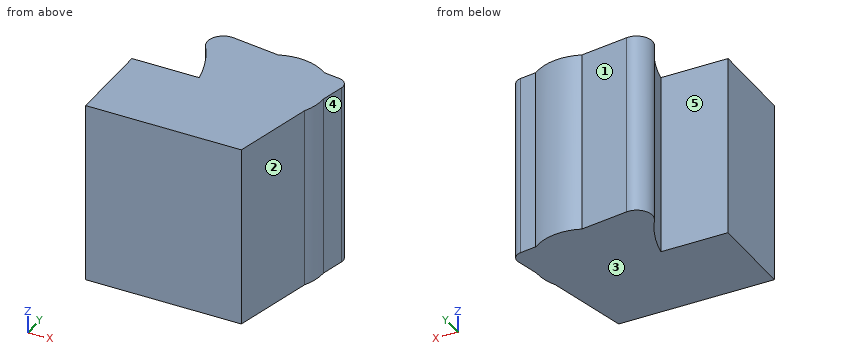
```python
from build123d import *

# Parameters (mm, degrees)
SKETCH_1_R                     = 27.60110162
EXTRUDE_1_DEPTH                = 50
SPLIT_BODIES_1_SURFACE_1_BACK  = 231.64
SPLIT_BODIES_1_SURFACE_1_DEPTH = 463.28
SPLIT_BODIES_1_SURFACE_2_BACK  = 231.64
SPLIT_BODIES_1_SURFACE_2_DEPTH = 463.28


with BuildPart() as part:
    # 草图1 → 凸台-拉伸1 (new, symmetric)
    with BuildSketch(Plane.XY):
        with Locations((126.841, 106.3205)):
            Circle(SKETCH_1_R)
        with BuildLine():
            Line((0, 29.556947787), (33.841128496, 29.556947787))
            Line((33.841128496, 29.556947787), (55.404404979, 43.133825573))
            Line((55.404404979, 43.133825573), (55.404404979, 95.897124924))
            Line((55.404404979, 95.897124924), (92.202864513, 95.897124924))
            ThreePointArc((92.202864513, 95.897124924), (88.266951773, 109.605982584), (81.786119565, 122.311217777))
            ThreePointArc((81.786119565, 122.311217777), (81.790702408, 131.54578908), (90.169806602, 135.427533672))
            Line((90.169806602, 135.427533672), (152.632483554, 126.981321854))
            ThreePointArc((152.632483554, 126.981321854), (156.573746893, 124.561834969), (157.437634447, 120.018579331))
            Line((157.437634447, 120.018579331), (140.698476255, 47.962391292))
            Line((140.698476255, 47.962391292), (125.156200351, 47.962391292))
            Line((125.156200351, 47.962391292), (116.770080258, 26.493923855))
            Line((116.770080258, 26.493923855), (133.542320443, 26.493923855))
            Line((133.542320443, 26.493923855), (144.001, 0))
            Line((144.001, 0), (0, 0))
            Line((0, 0), (0, 29.556947787))
        make_face()
    extrude(amount=EXTRUDE_1_DEPTH, both=True)


with BuildPart() as body_2:
    # Split Bodies 1: the piece behind the surface
    add(part.part)
    # Split Bodies 1 surface: a surface, the sketch's curves swept straight by 463.28 mm
    with BuildLine(Plane.XY.offset(50).offset(-SPLIT_BODIES_1_SURFACE_1_BACK), mode=Mode.PRIVATE) as split_bodies_1_surface_1_path:
        Line((125.156200351, 47.962391292), (37.921543342, 47.962391292))
    split_bodies_1_surface_1 = Shell.extrude(split_bodies_1_surface_1_path.wire(), (0 * SPLIT_BODIES_1_SURFACE_1_DEPTH, 0 * SPLIT_BODIES_1_SURFACE_1_DEPTH, 1 * SPLIT_BODIES_1_SURFACE_1_DEPTH))
    split(bisect_by=split_bodies_1_surface_1, keep=Keep.BOTTOM)


with BuildPart() as part_1:
    add(part.part)

    # Split Bodies 1: split by a surface, the side it looks to stays
    # Split Bodies 1 surface: a surface, the sketch's curves swept straight by 463.28 mm
    with BuildLine(Plane.XY.offset(50).offset(-SPLIT_BODIES_1_SURFACE_2_BACK), mode=Mode.PRIVATE) as split_bodies_1_surface_2_path:
        Line((125.156200351, 47.962391292), (37.921543342, 47.962391292))
    split_bodies_1_surface_2 = Shell.extrude(split_bodies_1_surface_2_path.wire(), (0 * SPLIT_BODIES_1_SURFACE_2_DEPTH, 0 * SPLIT_BODIES_1_SURFACE_2_DEPTH, 1 * SPLIT_BODIES_1_SURFACE_2_DEPTH))
    split(bisect_by=split_bodies_1_surface_2, keep=Keep.TOP)


solid = body_2.part
```
Part model, mm, in its own coordinate system. Face numbers are marked on the shaded views. A direction names the side the tool comes from. Coordinates: 2 decimals unless noted, no trailing zeros. Order: outer loops, then holes, each group sorted by start corner. A loop starts at its lowest first (then second) coordinate and runs counter-clockwise, first axis right, second up. Notation, with made-up numbers: (17, 65) - (44, 65) arc R33 ccw to (44, 98) - close; hole circle Ø10 at (76.5, 54.5). An arc over 180 degrees is marked (long way). Return JSON: item names as keys, results as strings. Group by question number.
Item 1: Drill centre lines: probe 1 along Y at (x, z) = (71, 13); probe 2 along Y at (x, z) = (128, -45); probe 3 along X at (y, z) = (92.5, 10.5). Where is each one in solid material? Low to high. Write a range as from..to.
Item 2: Pull direction Y, two halves, no side cores. Call the marked faces 3, 4 and 5: pulls with the +Y half, pulls with the -Y half, needs draft (parallel to the pull), parting line crosses it, or undercut.
Item 3: Cut at C-C (y = 71.5). List the corners of the cut face in (x, z), plus the area to 3 significant figures.
Item 4: Cut at B-B (x = 63). List the corners of the cut face in (y, z), plus the area to 3 significant figures.
Item 5: Cut at A-A (z = 4). List the corners of the cut face in (x, y).
Item 6: Pin check, flat tips, straight feed: pin 1 (4 mm diameter, centred on y = 123.5, z = 36, fed in from -X); pin 2 (8 mm diameter, centred on y = 74, z = 33.5, fed in from +X); pin 3 (2 mm diameter, centred on x = 119, z = 6.5, fed in from +Y). Stop position of each tip, or through.
Item 7: Which spindle directions (+Z, -Z, +X, -X, +Y, -Y) get a long thin tool onto all of the face, cutting with end or side? Do the marked faces 1 and 2. Say none if no direction does.
Check values:
{
 "1": {"probe 1": "y = 47.96..95.9", "probe 2": "y = 47.96..133.9", "probe 3": "x = 55.4..151.04"},
 "2": {"face 3": "needs draft", "face 4": "pulls with the -Y half", "face 5": "undercut"},
 "3": {"outline": "(55.4, -50) - (146.17, -50) - (146.17, 50) - (55.4, 50) - close", "area": "9,080 mm2"},
 "4": {"outline": "(47.96, -50) - (95.9, -50) - (95.9, 50) - (47.96, 50) - close", "area": "4,790 mm2"},
 "5": {"outline": "(55.4, 47.96) - (140.7, 47.96) - (151.27, 93.48) arc R27.6 ccw to (154.43, 107.08) - (157.44, 120.02) arc R5.72 ccw to (152.63, 126.98) - (143.68, 128.19) arc R27.6 ccw to (116.42, 131.88) - (90.17, 135.43) arc R8.58 ccw to (81.79, 122.31) arc R74.36 cw to (92.2, 95.9) - (55.4, 95.9) - close"},
 "6": {"pin 1": "stops at x = 80.56", "pin 2": "stops at x = 147.68", "pin 3": "stops at y = 133.06"},
 "7": {"face 1": "+Z, -Z, +Y", "face 2": "+Z, -Z, +X, -Y"}
}
